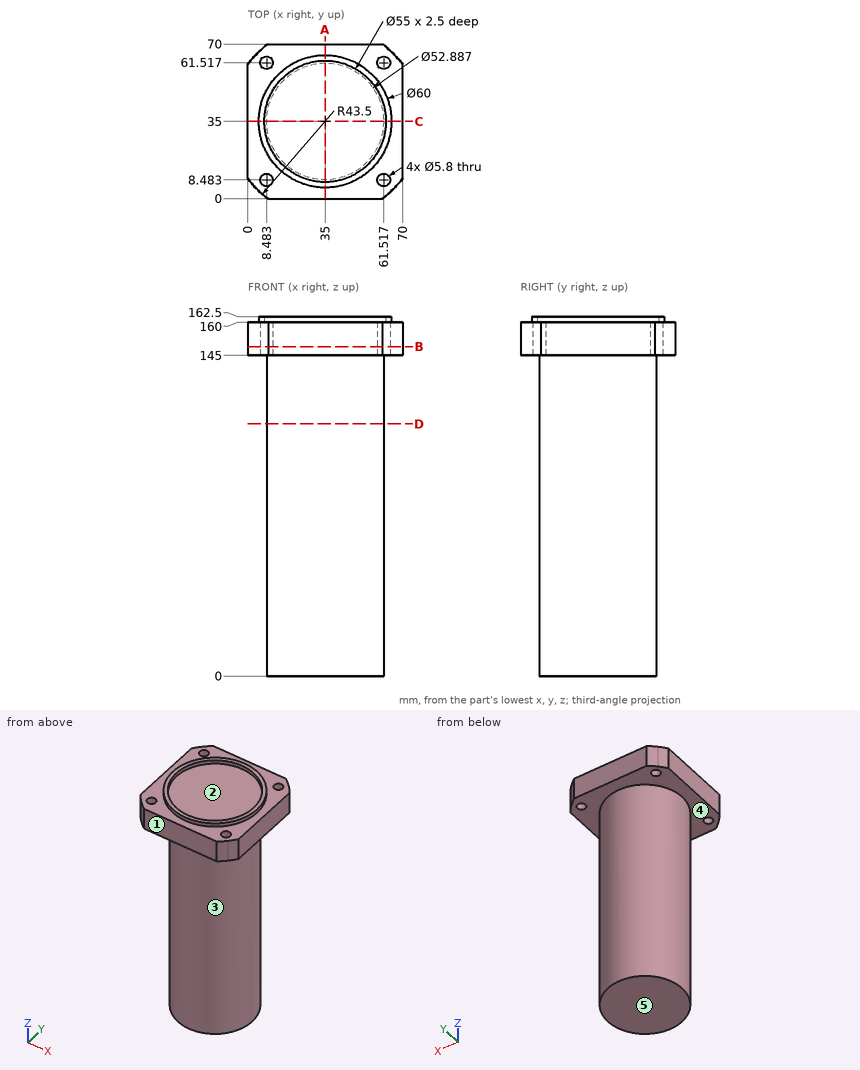
Drawing for the job (mm, zero at the part's lowest x, y, z). A direction names the side the tool comes from. Coordinates: 2 decimals unless noted, no trailing zeros. Loops run counter-clockwise (first coordinate to the right, second up) from the corner with the lowest first, then second, coordinate; pieces in that order, holes last. Notation, with made-up numbers: (77, 28.5) - (82, 28.5) arc R16 cw to (82, 51.5) - close; hole circle Ø8 at (13, -17). An arc over 180 degrees is marked (long way). Return JSON: item names as keys, results as strings.
1. Drop flat-ended pins along their axis: pin 1 (7.5 mm diameter, centred on x = 8.48, y = 61.52, fed in from -Z); pin 2 (1.5 mm diameter, centred on x = 55, z = 107, fed in from -Y); pin 3 (10 mm diameter, centred on x = 52, y = 40.5, fed in from +Z); pin 4 (5 mm diameter, centred on x = 10.5, y = 41, fed in from +Z). Give the stop position or say it passes through.
Result:
{"pin 1": "stops at z = 145", "pin 2": "stops at y = 16.87", "pin 3": "stops at z = 160", "pin 4": "stops at z = 162.5"}
2. Band-saw the part on B-B (z = 149). Give the cut face in (x, y), and give its area (3 significant figures).
Result:
{"outline": "(0, 9.17) arc R43.5 ccw to (9.17, 0) - (60.83, 0) arc R43.5 ccw to (70, 9.17) - (70, 60.83) arc R43.5 ccw to (60.83, 70) - (9.17, 70) arc R43.5 ccw to (0, 60.83) - close; hole circle Ø5.8 at (8.48, 8.48); hole circle Ø5.8 at (8.48, 61.52); hole circle Ø5.8 at (61.52, 8.48); hole circle Ø5.8 at (61.52, 61.52)", "area": "4,640 mm2"}
3. Band-saw the part on A-A (x = 35). Give the cut face in (y, z), and give its area (3 significant figures).
Result:
{"outline": "(0, 145) - (8.56, 145) - (8.56, 0) - (61.44, 0) - (61.44, 145) - (70, 145) - (70, 160) - (65, 160) - (65, 162.5) - (62.5, 162.5) - (62.5, 160) - (7.5, 160) - (7.5, 162.5) - (5, 162.5) - (5, 160) - (0, 160) - close", "area": "8,730 mm2"}
4. Band-saw the part on D-D (z = 114). Give the cut face in (x, y), and give its area (3 significant figures).
Result:
{"outline": "circle Ø52.89 at (35, 35)", "area": "2,200 mm2"}
5. Probe L1, parallel to Z at x = 64.5, y = 25; L2, parallel to Z at x = 14, y = 44; L3, parallel to Y at x = 35, z = 113.5. List the from-to ranges inside material, lowest first. Write a range as from..to.
Result:
{"L1": "z = 145..160", "L2": "z = 0..160", "L3": "y = 8.56..61.44"}
6. 3-axis set-ups, long thin cutter, end or side, ignore diameter. For the marked faces 4 and 5: which of +Z, -Z, +X, -X, +Y, -Y reach the whole face in a straight line?
Result:
{"face 4": "-Z", "face 5": "-Z, +X, -X, +Y, -Y"}
7. Mould opens along X. For the marked faces 1, 2 and 3 say: released by +X, released by -X, zero draft, split by the parting line, or undercut.
Result:
{"face 1": "zero draft", "face 2": "undercut", "face 3": "split by the parting line"}
